For this review, take the finished solid that the model builds, in its own axes (mm). Round coordinates to 2 decimals unless told otherwise and drop trailing zeros. Order: outer loops, then holes, each group sorted by start corner. A loop starts at its lowest first (then second) coordinate and runs counter-clockwise, first axis right, second up. Notation, with made-up numbers: (-2.5, 82.5) - (56.5, 82.5) arc R26 ccw to (56.5, 105.5) - close; hole circle Ø4 at (85.25, 72). An arc over 180 degrees is marked (long way). One line per item, written item: value.
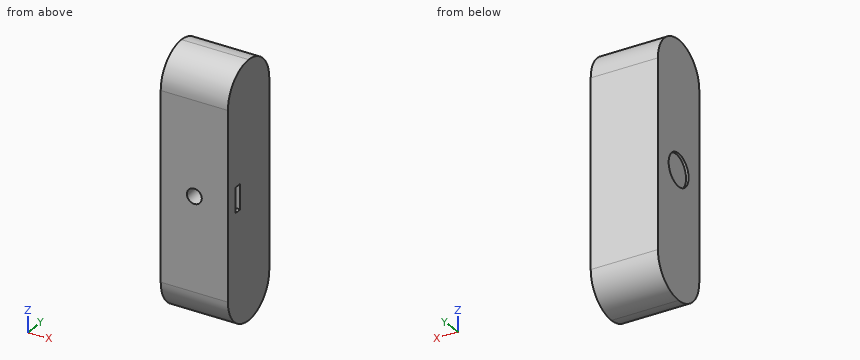
Autodesk Inventor part; units mm, degrees
ref_plane "YZ Plane" through (0, 0, 0) normal (1, 0, 0) x (0, 1, 0)
ref_plane "XZ Plane" through (0, 0, 0) normal (0, 1, 0) x (-1, 0, 0)
ref_plane "XY Plane" through (0, 0, 0) normal (0, 0, 1) x (1, 0, 0)
sketch "スケッチ1" plane through (0, 0, 0) normal (0, 1, 0) x (-1, 0, 0)
  line L0 (0, 0) -> (27, 0)
  line L1 (27, 0) -> (27, -102)
  line L2 (27, -102) -> (0, -102)
  line L3 (0, -102) -> (0, 0)
  dimension "d0" = 27
  dimension "d1" = 102
extrude "押し出し1" add sketch "スケッチ1" along normal blind 27
fillet "フィレット1" radius 13.5 4 edges at (-13.5, 27, 0) (-13.5, 0, 0) (-13.5, 27, -102) (-13.5, 0, -102)
sketch "スケッチ2" plane through (-27, 0, -88.5) normal (-1, 0, 0) x (0, 0, 1)
  line L0 (0, 27) -> (75, 27)
  line L1 (37.5, 27) -> (37.5, 0)
  line L2 (0, 0) -> (75, 0)
  circle A0 centre (37.5, 13.5) radius 6.5
  point P0 (88.5, 0)
  dimension "d5" = 13
extrude "押し出し2" cut sketch "スケッチ2" against normal blind 1
sketch "スケッチ3" plane through (0, 0, 0) normal (0, -1, 0) x (1, 0, 0)
  line L0 (-27, -88.5) -> (-27, -13.5)
  line L1 (-27, -51) -> (0, -51)
  line L2 (0, -13.5) -> (0, -88.5)
  point P0 (0, 0)
  point P1 (-13.5, -51)
hole "穴1" at (-13.5, 0, -51) direction (0, 1, 0) diameter 6 depth 8 tip angle 118
sketch "スケッチ4" plane through (0, 0, -13.5) normal (1, 0, 0) x (0, 0, -1)
  line L0 (32.5, 8) -> (42.5, 8)
  line L1 (42.5, 8) -> (42.5, 5)
  line L2 (42.5, 5) -> (32.5, 5)
  line L3 (32.5, 5) -> (32.5, 8)
  line L4 (0, 0) -> (75, 0)
  point P0 (-13.5, 0)
  point P1 (37.5, 0)
  point P2 (37.5, 5)
  dimension "d15" = 10
  dimension "d16" = 3
  dimension "d17" = 5
  dimension "d18" = 0
extrude "押し出し3" cut sketch "スケッチ4" against normal blind 5
properties part number "camera" material "ABS プラスチック"
Item 1: Wall thickness on line 1 (X direction, y = 2.75, z = -51); line 2 (X direction, y = 5.75, z = -51); line 3 (Z direction, x = -26.55, y = 13.5): over which ranges is each line inside the solid? List them lowest first.
Returned:
line 1: -27 to -16.5, -10.5 to 0
line 2: -27 to -16.5, -10.5 to -5
line 3: -102 to -57.5, -44.5 to 0
Item 2: Take a section at B-B (y = 24.75). Write out the cut boundary in (x, z), plus the area to 3 significant figures.
Returned:
outline: (-27, -95.96) - (0, -95.96) - (0, -6.04) - (-27, -6.04) - close
area: 2,430 mm^2
Item 3: For P1, Ø1.5, axis at x = -3.5, y = 6, coming from the -Z side; P2, Ø4, axis at y = 12.5, z = -52.5, coming from the -X side; P3, Ø1.5, axis at x = -14.5, y = 9, coming from the -Z side, all flat-tipped, find the tip position at first contact; note any pin that passes through.
Returned:
P1: z = -100.19
P2: x = -26
P3: z = -101.47
